from build123d import *

# Parameters (mm, degrees)
EXTRUDE_4_DEPTH     = 3
SKETCH_5_R          = 3.5
EXTRUDE_6_DEPTH     = 4.5
FILLET_1_R          = 0.5
CUT_EXTRUDE_1_DEPTH = 8.5


with BuildPart() as part:
    # 草图4 → 凸台-拉伸4 (new body)
    with BuildSketch(Plane.XY):
        with BuildLine():
            ThreePointArc((8.536063079, 0.007574004), (7.787120491, 0.307636704), (6.986931627, 0.410837493))
            ThreePointArc((6.986931627, 0.410837493), (6.952112765, 0.808782481), (6.894647301, 1.204092849))
            ThreePointArc((6.894647301, 1.204092849), (7.649774364, 1.488233206), (8.309831075, 1.95221355))
            ThreePointArc((8.309831075, 1.95221355), (8.220185959, 2.300646222), (8.115937918, 2.644991862))
            ThreePointArc((8.115937918, 2.644991862), (7.310926717, 2.698932461), (6.518011085, 2.549810286))
            ThreePointArc((6.518011085, 2.549810286), (6.361924616, 2.91751884), (6.18511409, 3.275723537))
            ThreePointArc((6.18511409, 3.275723537), (6.815478405, 3.77930417), (7.29985183, 4.424544441))
            ThreePointArc((7.29985183, 4.424544441), (7.106922641, 4.72822174), (6.901368208, 5.023499488))
            ThreePointArc((6.901368208, 5.023499488), (6.119088497, 4.826037904), (5.411062205, 4.439189883))
            ThreePointArc((5.411062205, 4.439189883), (5.148986959, 4.740668128), (4.870138818, 5.026703581))
            ThreePointArc((4.870138818, 5.026703581), (5.314035933, 5.70043051), (5.575312226, 6.463770094))
            ThreePointArc((5.575312226, 6.463770094), (5.297984218, 6.69296597), (5.011244492, 6.910271984))
            ThreePointArc((5.011244492, 6.910271984), (4.328271261, 6.480737132), (3.774440855, 5.894030644))
            ThreePointArc((3.774440855, 5.894030644), (3.432030584, 6.099767788), (3.078440426, 6.285634856))
            ThreePointArc((3.078440426, 6.285634856), (3.292418599, 7.063558994), (3.305022217, 7.870276894))
            ThreePointArc((3.305022217, 7.870276894), (2.970442186, 8.002556058), (2.63058525, 8.12061891))
            ThreePointArc((2.63058525, 8.12061891), (2.113772678, 7.501056656), (1.768350936, 6.77192262))
            ThreePointArc((1.768350936, 6.77192262), (1.379123142, 6.861779679), (0.985402836, 6.929284397))
            ThreePointArc((0.985402836, 6.929284397), (0.948516393, 7.735257109), (0.711213605, 8.506386157))
            ThreePointArc((0.711213605, 8.506386157), (0.352132577, 8.528800203), (-0.007574004, 8.536063079))
            ThreePointArc((-0.007574004, 8.536063079), (-0.307636703, 7.787120491), (-0.410837493, 6.986931627))
            ThreePointArc((-0.410837493, 6.986931627), (-0.808782481, 6.952112765), (-1.204092849, 6.894647301))
            ThreePointArc((-1.204092849, 6.894647301), (-1.488233206, 7.649774364), (-1.95221355, 8.309831075))
            ThreePointArc((-1.95221355, 8.309831075), (-2.300646222, 8.220185959), (-2.644991862, 8.115937918))
            ThreePointArc((-2.644991862, 8.115937918), (-2.698932461, 7.310926717), (-2.549810286, 6.518011085))
            ThreePointArc((-2.549810286, 6.518011085), (-2.91751884, 6.361924616), (-3.275723537, 6.18511409))
            ThreePointArc((-3.275723537, 6.18511409), (-3.77930417, 6.815478405), (-4.424544441, 7.29985183))
            ThreePointArc((-4.424544441, 7.29985183), (-4.72822174, 7.106922641), (-5.023499488, 6.901368208))
            ThreePointArc((-5.023499488, 6.901368208), (-4.826037904, 6.119088497), (-4.439189882, 5.411062205))
            ThreePointArc((-4.439189882, 5.411062205), (-4.740668128, 5.148986959), (-5.026703581, 4.870138818))
            ThreePointArc((-5.026703581, 4.870138818), (-5.70043051, 5.314035933), (-6.463770094, 5.575312226))
            ThreePointArc((-6.463770094, 5.575312226), (-6.69296597, 5.297984218), (-6.910271984, 5.011244492))
            ThreePointArc((-6.910271984, 5.011244492), (-6.480737132, 4.328271262), (-5.894030644, 3.774440855))
            ThreePointArc((-5.894030644, 3.774440855), (-6.099767788, 3.432030584), (-6.285634856, 3.078440426))
            ThreePointArc((-6.285634856, 3.078440426), (-7.063558994, 3.292418599), (-7.870276894, 3.305022217))
            ThreePointArc((-7.870276894, 3.305022217), (-8.002556058, 2.970442186), (-8.12061891, 2.63058525))
            ThreePointArc((-8.12061891, 2.63058525), (-7.501056656, 2.113772678), (-6.77192262, 1.768350936))
            ThreePointArc((-6.77192262, 1.768350936), (-6.861779679, 1.379123142), (-6.929284397, 0.985402836))
            ThreePointArc((-6.929284397, 0.985402836), (-7.735257109, 0.948516393), (-8.506386157, 0.711213605))
            ThreePointArc((-8.506386157, 0.711213605), (-8.528800203, 0.352132577), (-8.536063079, -0.007574004))
            ThreePointArc((-8.536063079, -0.007574004), (-7.787120492, -0.307636703), (-6.986931627, -0.410837493))
            ThreePointArc((-6.986931627, -0.410837493), (-6.952112765, -0.808782481), (-6.894647301, -1.204092849))
            ThreePointArc((-6.894647301, -1.204092849), (-7.649774364, -1.488233206), (-8.309831076, -1.95221355))
            ThreePointArc((-8.309831076, -1.95221355), (-8.220185959, -2.300646222), (-8.115937918, -2.644991862))
            ThreePointArc((-8.115937918, -2.644991862), (-7.310926717, -2.698932461), (-6.518011085, -2.549810286))
            ThreePointArc((-6.518011085, -2.549810286), (-6.361924616, -2.91751884), (-6.18511409, -3.275723537))
            ThreePointArc((-6.18511409, -3.275723537), (-6.815478405, -3.77930417), (-7.29985183, -4.424544441))
            ThreePointArc((-7.29985183, -4.424544441), (-7.106922641, -4.72822174), (-6.901368208, -5.023499488))
            ThreePointArc((-6.901368208, -5.023499488), (-6.119088498, -4.826037904), (-5.411062205, -4.439189883))
            ThreePointArc((-5.411062205, -4.439189883), (-5.148986959, -4.740668128), (-4.870138818, -5.026703582))
            ThreePointArc((-4.870138818, -5.026703582), (-5.314035933, -5.70043051), (-5.575312227, -6.463770094))
            ThreePointArc((-5.575312227, -6.463770094), (-5.297984218, -6.69296597), (-5.011244492, -6.910271984))
            ThreePointArc((-5.011244492, -6.910271984), (-4.328271262, -6.480737132), (-3.774440855, -5.894030644))
            ThreePointArc((-3.774440855, -5.894030644), (-3.432030584, -6.099767789), (-3.078440426, -6.285634856))
            ThreePointArc((-3.078440426, -6.285634856), (-3.292418599, -7.063558994), (-3.305022217, -7.870276894))
            ThreePointArc((-3.305022217, -7.870276894), (-2.970442186, -8.002556058), (-2.63058525, -8.12061891))
            ThreePointArc((-2.63058525, -8.12061891), (-2.113772678, -7.501056656), (-1.768350936, -6.77192262))
            ThreePointArc((-1.768350936, -6.77192262), (-1.379123142, -6.861779679), (-0.985402836, -6.929284397))
            ThreePointArc((-0.985402836, -6.929284397), (-0.948516393, -7.735257109), (-0.711213605, -8.506386157))
            ThreePointArc((-0.711213605, -8.506386157), (-0.352132577, -8.528800203), (0.007574004, -8.536063079))
            ThreePointArc((0.007574004, -8.536063079), (0.307636704, -7.787120491), (0.410837493, -6.986931627))
            ThreePointArc((0.410837493, -6.986931627), (0.808782481, -6.952112765), (1.204092849, -6.894647301))
            ThreePointArc((1.204092849, -6.894647301), (1.488233206, -7.649774364), (1.95221355, -8.309831075))
            ThreePointArc((1.95221355, -8.309831075), (2.300646222, -8.220185959), (2.644991862, -8.115937918))
            ThreePointArc((2.644991862, -8.115937918), (2.698932461, -7.310926717), (2.549810286, -6.518011085))
            ThreePointArc((2.549810286, -6.518011085), (2.91751884, -6.361924616), (3.275723537, -6.18511409))
            ThreePointArc((3.275723537, -6.18511409), (3.77930417, -6.815478405), (4.424544441, -7.29985183))
            ThreePointArc((4.424544441, -7.29985183), (4.72822174, -7.106922641), (5.023499488, -6.901368208))
            ThreePointArc((5.023499488, -6.901368208), (4.826037904, -6.119088497), (4.439189883, -5.411062205))
            ThreePointArc((4.439189883, -5.411062205), (4.740668128, -5.148986959), (5.026703582, -4.870138818))
            ThreePointArc((5.026703582, -4.870138818), (5.70043051, -5.314035933), (6.463770094, -5.575312226))
            ThreePointArc((6.463770094, -5.575312226), (6.69296597, -5.297984218), (6.910271984, -5.011244492))
            ThreePointArc((6.910271984, -5.011244492), (6.480737132, -4.328271261), (5.894030644, -3.774440855))
            ThreePointArc((5.894030644, -3.774440855), (6.099767788, -3.432030584), (6.285634856, -3.078440425))
            ThreePointArc((6.285634856, -3.078440425), (7.063558994, -3.292418599), (7.870276894, -3.305022217))
            ThreePointArc((7.870276894, -3.305022217), (8.002556058, -2.970442186), (8.12061891, -2.63058525))
            ThreePointArc((8.12061891, -2.63058525), (7.501056656, -2.113772678), (6.77192262, -1.768350936))
            ThreePointArc((6.77192262, -1.768350936), (6.861779679, -1.379123142), (6.929284397, -0.985402836))
            ThreePointArc((6.929284397, -0.985402836), (7.735257109, -0.948516393), (8.506386157, -0.711213605))
            ThreePointArc((8.506386157, -0.711213605), (8.528643141, -0.355916321), (8.536066439, 0))
            ThreePointArc((8.536066439, 0), (8.536065599, 0.003787002), (8.536063079, 0.007574004))
        make_face()
    extrude(amount=EXTRUDE_4_DEPTH)

    # 草图5 → 凸台-拉伸6 (add)
    with BuildSketch(Plane.XY.offset(3)):
        Circle(SKETCH_5_R)
    extrude(amount=EXTRUDE_6_DEPTH)

    # 圆角1
    fillet_1_edges = [part.edges().sort_by_distance(p)[0] for p in [
        (-3.5, 0, 7.5),
    ]]
    fillet(fillet_1_edges, radius=FILLET_1_R)

    # 草图8 → 切除-拉伸1 (cut, through all)
    with BuildSketch(Plane(origin=(0, 0, 0), x_dir=(-1, 0, 0), z_dir=(0, 0, -1))):
        with BuildLine():
            Line((0.342458427, -1.460384273), (1.413290623, 0.50260284))
            ThreePointArc((1.413290623, 0.50260284), (-1.316811787, 0.718336075), (0.342458427, -1.460384273))
        make_face()
    extrude(amount=-CUT_EXTRUDE_1_DEPTH, mode=Mode.SUBTRACT)


solid = part.part
The model under review builds one solid part; all positions refer to its coordinate system, in mm. A direction names the side the tool comes from. Round coordinates to 2 decimals unless told otherwise and drop trailing zeros. Write each loop counter-clockwise with the first axis right and the second up, starting at its lowest first coordinate (ties: lowest second). Pieces come first, ordered by that corner, then holes. Notation, with made-up numbers: (-12, -13.75) - (46, -13.75) arc R20 ccw to (46, 5.25) - close; hole circle Ø2 at (-36, -7). An arc over 180 degrees is marked (long way). One line per item, written item: value. Start each with the question number.
1. Machinability: for faces 4 (the face through (0.305, -7.798, 1.479)), 5 (the face through (6.808, 3.771, 1.479)), 6 (the face through (-3.29, -7.05, 1.48)), which of the approach directions +Z, -Z, +X, -X, +Y, -Y give a long, thin tool a straight path to every point of the face, cutting with its end or side? Answer none if there is none.
2. Consider section A-A on y = 4. Write out the cut boundary in (x, z), and give its area (3 significant figures).
3. To check wall thickness, follow L1, parallel to Y at x = 0, z = 3.75; L2, parallel to Z at x = 3.75, y = 3.5; L3, parallel to X at y = 0.25, z = 3.75. State the ranges of each line that lie inside material, in increasing order. Write a range as from..to.
4. The part is to be moulded in two halves that separate along Y. For faces 1 (the face through (-5.31, -5.69, 1.48)), 2 (the face through (2.12, 7.51, 1.48)), 3 (the face through (-1.4, 0, 7.5)), say which applies: released by +Y, released by -Y, zero draft, split by the parting line, or undercut.
Checks:
1. face 4: +Z, -Z, -Y
1. face 5: +Z, -Z, +X
1. face 6: +Z, -Z
2. outline: (-6.17, 0) - (7.01, 0) - (7.01, 3) - (-6.17, 3) - close
2. area: 39.5 mm^2
3. L1: y = -3.5..-1.5, 1.5..3.5
3. L2: z = 0..3
3. L3: x = -3.49..-1.28, 1.48..3.49
4. face 1: undercut
4. face 2: released by +Y
4. face 3: zero draft
